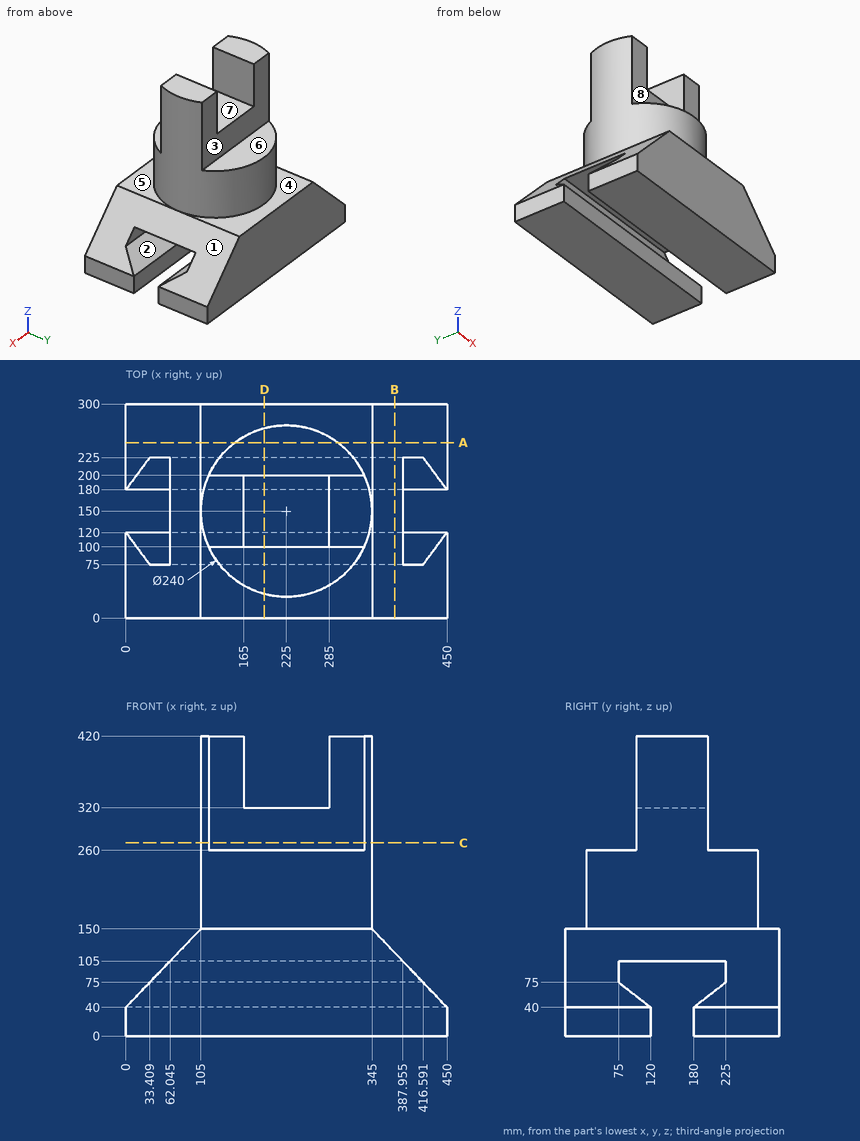
Verification items for this drawing (mm, ordinates from the low corner). A direction names the side the tool comes from. Round coordinates to 2 decimals unless told otherwise and drop trailing zeros. Write each loop counter-clockwise with the first axis right and the second up, starting at its lowest first coordinate (ties: lowest second). Pieces come first, ordered by that corner, then holes. Notation, with made-up numbers: M 71,44.5 L 90,44.5 A17 ccw 90,50.5 Z; hole C 77.25,57 d2. An arc over 180 degrees is marked long. Write item = value, one per line. Start each with the question number.
1. Section check B-B, the plane x = 376.5. Record the cut outline in (y, z), then the cut area to 3 significant figures.
2. Tool access check on the marked faces 4, 5, 6, 7 and 8. Record the directions out of +Z, -Z, +X, -X, +Y, -Y that give a thin tool (end or side, any length) a straight path to the whole face; none if there is none.
3. Section check C-C, the plane z = 270.5. Record the cut outline in (x, y).
4. Release check for a two-part mould opening along Y. For the marked faces 1, 2 and 3 record: pulls with the +Y half, pulls with the -Y half, needs draft (parallel to the pull), parting line crosses it, or undercut.
5. Gauge pin test, flat ends, axial feed: pin 1 (5 mm diameter, centred on x = 66.5, y = 174.5, fed in from -Z); pin 2 (12 mm diameter, centred on y = 209, z = 66.5, fed in from -X); pin 3 (6 mm diameter, centred on x = 88, y = 191.5, fed in from +Z) (1 decimal); pin 4 (20 mm diameter, centred on x = 323.5, z = 26, fed in from -Y). Record the tip position at first contact, or that the pin passes through.
6. Scan lines: line 1 (Y direction, x = 308.5, z = 17); line 2 (Z direction, x = 111.5, y = 270); line 3 (X direction, y = 163, z = 340.5). Record each from-to range of solid material in increasing order. Write a range as [from, to].
7. Section check A-A, the plane y = 246. Record the cut outline in (x, z).
8. Section check D-D, the plane x = 194. Record the cut outline in (y, z).
Results found:
q1.outline = M 0,0 L 120,0 L 120,40 L 75,75 L 75,105 L 225,105 L 225,75 L 180,40 L 180,0 L 300,0 L 300,117 L 0,117 Z
q1.area = 24,500 mm^2
q2.face_4 = +Z, +Y
q2.face_5 = +Z, -Y
q2.face_6 = +Z, +X, -X, +Y
q2.face_7 = +Z, +Y, -Y
q2.face_8 = +Z, +X, -X, -Y
q3.outline = M 115.91,100 L 334.09,100 A120 ccw 334.09,200 L 115.91,200 A120 ccw Z
q4.face_1 = needs draft
q4.face_2 = undercut
q4.face_3 = pulls with the +Y half
q5.pin_1 = 105
q5.pin_2 = 19.57
q5.pin_3 = 135.3
q5.pin_4 = 0
q6.line_1 = [0, 120], [180, 300]
q6.line_2 = [0, 150]
q6.line_3 = [105.71, 165], [285, 344.29]
q7.outline = M 0,0 L 450,0 L 450,40 L 345,150 L 297,150 L 297,260 L 153,260 L 153,150 L 105,150 L 0,40 Z
q8.outline = M 0,0 L 120,0 L 120,40 L 75,75 L 75,105 L 225,105 L 225,75 L 180,40 L 180,0 L 300,0 L 300,150 L 265.93,150 L 265.93,260 L 200,260 L 200,320 L 100,320 L 100,260 L 34.07,260 L 34.07,150 L 0,150 Z
